from build123d import *

# Parameters (mm, degrees)
BOSS_EXTRUDE1_DEPTH = 4.08
CUT_EXTRUDE1_DEPTH  = 0.3
CUT_EXTRUDE2_DEPTH  = 0.3


with BuildPart() as part:
    # Sketch1 → Boss-Extrude1 (new body)
    with BuildSketch(Plane(origin=(0, 0, 0), x_dir=(1, 0, 0), z_dir=(0, 1, 0))):
        Polygon((-0.15, 0), (-0.15, 0.287479127), (-10.410512779, 3.278145873), (-10.326564075, 3.56616083), (0.15, 0.512520873), (0.15, 0), align=None)
    extrude(amount=BOSS_EXTRUDE1_DEPTH)

    # Sketch2 → Cut-Extrude1 (cut)
    with BuildSketch(Plane(origin=(0.149434274, 0, -0.512685767), x_dir=(-0.9600498543859305, 0, -0.2798290140309858), z_dir=(0.2798290140309858, 0, -0.9600498543859306))):
        with BuildLine():
            Line((0.969410732, 1.39), (7.969410732, 1.39))
            ThreePointArc((7.969410732, 1.39), (8.619410732, 2.04), (7.969410732, 2.69))
            Line((7.969410732, 2.69), (0.969410732, 2.69))
            Line((0.969410732, 2.69), (0.969410732, 1.39))
        make_face()
    extrude(amount=-CUT_EXTRUDE1_DEPTH, mode=Mode.SUBTRACT)

    # Sketch3 → Cut-Extrude2 (cut)
    with BuildSketch(Plane(origin=(0.149434274, 0, -0.512685767), x_dir=(-0.9600498543859305, 0, -0.2798290140309858), z_dir=(0.2798290140309858, 0, -0.9600498543859306))):
        with BuildLine():
            Line((5.561931606, 4.08), (6.261931606, 4.08))
            ThreePointArc((6.261931606, 4.08), (5.911931606, 3.73), (5.561931606, 4.08))
        make_face()
        with BuildLine():
            Line((5.561931606, 0), (6.261931606, 0))
            ThreePointArc((6.261931606, 0), (5.911931606, 0.35), (5.561931606, 0))
        make_face()
    extrude(amount=-CUT_EXTRUDE2_DEPTH, mode=Mode.SUBTRACT)


solid = part.part
Can you work these out from the model? Positions are in its coordinate system, mm. Round coordinates to 2 decimals unless told otherwise and drop trailing zeros. Write each loop counter-clockwise with the first axis right and the second up, starting at its lowest first coordinate (ties: lowest second). Pieces come first, ordered by that corner, then holes. Notation, with made-up numbers: (80.5, 82.5) - (93.5, 82.5) arc R10 ccw to (93.5, 94.5) - close; hole circle Ø2 at (28, 17). An arc over 180 degrees is marked (long way). Write each question's results on one line, items separated by ' | '. Start each with the question number.
1) Suppose I cut it at A-A (x = -2.5). List the corners of the cut face in (y, z) for me, and give its area (3 significant figures).
2) Please list where these lines run through material, in increasing order: line 1 (Y direction, x = -3.5, z = -1.45); line 2 (Z direction, x = -1, y = 2.95); line 3 (Z direction, x = -1.5, y = 0.55).
3) For pin 1 Ø1.5 at (x, y) = (-5, 2) entering from -Z; pin 2 Ø2 at (x, y) = (-3.5, 3.5) entering from +Z, each with a flat end and sliding along its axis, tell me the tip position at first contact or that it passes through.
4) Suppose I cut it at B-B (z = -1.2). List the corners of the cut face in (x, y) for me.
5) Suppose I cut it at D-D (y = 3.55). List the corners of the cut face in (x, z) for me, and give its area (3 significant figures).
6) Suppose I cut it at C-C (y = 2.1). List the corners of the cut face in (x, z) for me.
Here are the results:
1) outline: (0, -1.28) - (1.39, -1.28) - (1.39, -0.97) - (0, -0.97) - close; (2.69, -1.28) - (4.08, -1.28) - (4.08, -0.97) - (2.69, -0.97) - close | area: 0.869 mm2
2) line 1: y = 0 to 1.39, 2.69 to 4.08 | line 2: z = -0.85 to -0.54 | line 3: z = -0.99 to -0.68
3) pin 1: stops at z = -2.14 | pin 2: stops at z = -0.97
4) outline: (-3.28, 0) - (-2.21, 0) - (-2.21, 1.39) - (-3.28, 1.39) - close; (-3.28, 2.69) - (-2.21, 2.69) - (-2.21, 4.08) - (-3.28, 4.08) - close
5) outline: (-10.41, -3.28) - (-10.33, -3.57) - (0.15, -0.51) - (0.15, 0) - (-0.15, 0) - (-0.15, -0.29) - close | area: 3.36 mm2
6) outline: (-10.41, -3.28) - (-10.33, -3.57) - (-8.12, -2.92) - (-8.21, -2.64) - close; (-0.87, -0.5) - (-0.78, -0.78) - (0.15, -0.51) - (0.15, 0) - (-0.15, 0) - (-0.15, -0.29) - close
